Part model, mm, in its own coordinate system. A direction names the side the tool comes from. Give positions to 0.01 mm unless a question says otherwise; leave off trailing zeros. Write each loop counter-clockwise with the first axis right and the second up, starting at its lowest first coordinate (ties: lowest second). Pieces come first, ordered by that corner, then holes.
Autodesk Inventor part; units mm, degrees
ref_plane "YZ Plane" through (0, 0, 0) normal (1, 0, 0) x (0, 1, 0)
ref_plane "XZ Plane" through (0, 0, 0) normal (0, 1, 0) x (-1, 0, 0)
ref_plane "XY Plane" through (0, 0, 0) normal (0, 0, 1) x (1, 0, 0)
sketch "Sketch4" plane through (0, 0, 0) normal (0, 0, 1) x (1, 0, 0)
  line L0 (0, 0) -> (150, 0)
  line L1 (150, 0) -> (150, 150)
  line L2 (150, 150) -> (0, 150)
  line L3 (0, 150) -> (0, 0)
  dimension "d34" = 150
  dimension "d35" = 150
extrude "Extrusion4" add sketch "Sketch4" along normal blind 10
sketch "Sketch5" plane through (0, 0, 10) normal (0, 0, 1) x (1, 0, 0)
  line L0 (10, 10) -> (140, 10)
  line L1 (140, 10) -> (140, 140)
  line L2 (140, 140) -> (10, 140)
  line L3 (10, 140) -> (10, 10)
  point P0 (0, 0)
  dimension "d38" = 130
  dimension "d39" = 130
extrude "Extrusion5" cut sketch "Sketch5" against normal blind 2
sketch "Sketch6" plane through (0, 0, 0) normal (0, 0, -1) x (-1, 0, 0)
  circle A0 centre (-75, 75) radius 14.35
  circle A1 centre (-75, 75) radius 17.15
  line L0 (-147.5, 2.5) -> (-142.5, 2.5)
  line L1 (-142.5, 2.5) -> (-142.5, 7.5)
  line L2 (-142.5, 7.5) -> (-147.5, 7.5)
  line L3 (-147.5, 7.5) -> (-147.5, 2.5)
  line L4 (-2.5, 2.5) -> (-7.5, 2.5)
  line L5 (-7.5, 2.5) -> (-7.5, 7.5)
  line L6 (-7.5, 7.5) -> (-2.5, 7.5)
  line L7 (-2.5, 7.5) -> (-2.5, 2.5)
  line L8 (-147.5, 147.5) -> (-142.5, 147.5)
  line L9 (-142.5, 147.5) -> (-142.5, 142.5)
  line L10 (-142.5, 142.5) -> (-147.5, 142.5)
  line L11 (-147.5, 142.5) -> (-147.5, 147.5)
  line L12 (-2.5, 147.5) -> (-7.5, 147.5)
  line L13 (-7.5, 147.5) -> (-7.5, 142.5)
  line L14 (-7.5, 142.5) -> (-2.5, 142.5)
  line L15 (-2.5, 142.5) -> (-2.5, 147.5)
  point P0 (0, 0)
  dimension "d42" = 28.7
  dimension "d43" = 34.3
  dimension "d46" = 5
  dimension "d47" = 5
  dimension "d48" = 5
  dimension "d49" = 5
  dimension "d50" = 5
  dimension "d51" = 5
  dimension "d52" = 5
  dimension "d53" = 5
extrude "Extrusion7" cut sketch "Sketch6" against normal blind 5
sketch "Sketch7" plane through (0, 0, 8) normal (0, 0, 1) x (1, 0, 0)
  line L0 (47.5, 102.5) -> (102.5, 102.5)
  line L1 (102.5, 102.5) -> (102.5, 47.5)
  line L2 (102.5, 47.5) -> (47.5, 47.5)
  line L3 (47.5, 47.5) -> (47.5, 102.5)
  point P0 (0, 0)
  dimension "d58" = 55
  dimension "d59" = 55
extrude "Extrusion8" cut sketch "Sketch7" against normal blind 2
properties part number "Elbow_Parallel_Joint"
1) Two-plate mould, pull along Y, no slides. Class faces 1 (the face through (76, 150, 5)), 2 (the face through (5, 5, 5)), 3 (the face through (141, 76, 10)), 4 (the face through (74, 0, 5)): +Y half, -Y half, draft (parallel to the pull), parting line (faces both ways), or undercut.
Answers follow:
face 1: +Y half
face 2: undercut
face 3: draft
face 4: -Y half
2) Wall check: L1, parallel to Y at x = 75, z = 2.65; L2, parallel to X at y = 23, z = 9.5. Give the ranges that are in metal, low to high.
Answers follow:
L1: y = 0 to 57.85, 60.65 to 89.35, 92.15 to 150
L2: x = 0 to 10, 140 to 150
3) Pin check, flat tips, straight feed: pin 1 Ø4 at (x, z) = (144, 1.5) entering from -Y; pin 2 Ø1.5 at (x, y) = (144.5, 144.5) entering from -Z. Stop position of each tip, or through.
Answers follow:
pin 1: stops at y = 0
pin 2: stops at z = 5
4) 3-axis set-ups, long thin cutter, end or side, ignore diameter. For faces 5 (the face through (145, 147.5, 2)), 6 (the face through (0, 76, 5)), 7 (the face through (45, 76, 8)): which of +Z, -Z, +X, -X, +Y, -Y reach the whole face in a straight line?
Answers follow:
face 5: -Z
face 6: +Z, -Z, -X, +Y, -Y
face 7: +Z
5) Saw through at B-B, the plane y = 75. Write the cut outline in (x, z), then the cut area to 3 significant figures.
Answers follow:
outline: (0, 0) - (57.85, 0) - (57.85, 5) - (60.65, 5) - (60.65, 0) - (89.35, 0) - (89.35, 5) - (92.15, 5) - (92.15, 0) - (150, 0) - (150, 10) - (140, 10) - (140, 8) - (102.5, 8) - (102.5, 6) - (47.5, 6) - (47.5, 8) - (10, 8) - (10, 10) - (0, 10) - close
area: 1,100 mm2
6) Saw through at C-C, the plane x = 36. Write the cut outline in (y, z).
Answers follow:
outline: (0, 0) - (150, 0) - (150, 10) - (140, 10) - (140, 8) - (10, 8) - (10, 10) - (0, 10) - close
7) Saw through at A-A, the plane z = 2.5. Write the cut outline in (x, y).
Answers follow:
outline: (0, 0) - (150, 0) - (150, 150) - (0, 150) - close; circle Ø28.7 at (75, 75); hole (2.5, 2.5) - (7.5, 2.5) - (7.5, 7.5) - (2.5, 7.5) - close; hole (2.5, 142.5) - (7.5, 142.5) - (7.5, 147.5) - (2.5, 147.5) - close; hole circle Ø34.3 at (75, 75); hole (142.5, 2.5) - (147.5, 2.5) - (147.5, 7.5) - (142.5, 7.5) - close; hole (142.5, 142.5) - (147.5, 142.5) - (147.5, 147.5) - (142.5, 147.5) - close
